Build history of the part. All positions in model axes, mm. A direction names the side the tool comes from. Give positions to 0.01 mm unless a question says otherwise; leave off trailing zeros. Order: outer loops, then holes, each group sorted by start corner. A loop starts at its lowest first (then second) coordinate and runs counter-clockwise, first axis right, second up. Notation, with made-up numbers: (84, -39) - (123, -39) arc R18 ccw to (123, -6) - close; hole circle Ø11 at (43, 70.5). An arc over 180 degrees is marked (long way). Use a Markdown table: item, result. Add a question column.
(1) Flat gauge pins, fed straight in: pin 1 (4 mm diameter, centred on y = 16.5, z = 25, fed in from -X); pin 2 (8 mm diameter, centred on x = 24.73, z = 80, fed in from +Y); pin 3 (11.5 mm diameter, centred on x = 24.73, z = 10, fed in from +Y); pin 4 (4 mm diameter, centred on x = -24.73, z = 10, fed in from -Y). Where does each tip first touch, or does it go through?
(2) Slice it at B-B (z = 31.5). Write the cut outline in (x, y), then the cut area to 3 significant figures.
(3) Wall check: line 1 (Z direction, x = -26, y = 11.5); line 2 (X direction, y = 24, z = 5); line 3 (X direction, y = 21.75, z = 5). Give the ranges that are in metal, low to high.
(4) Slice it at C-C (y = 8.5). Write the cut outline in (x, z).
(5) Which spindle directions (+Z, -Z, +X, -X, +Y, -Y) get a long thin tool onto all of the face, cutting with end or side? Do faces 4 (the face through (0, 19, 0)), 5 (the face through (-19.77, 11.97, 80.65)), 6 (the face through (-12.5, 19, 45)). Say none if no direction does.
(6) Slice it at D-D (z = 10). Write the cut outline in (x, y), then the cut area to 3 significant figures.
(7) Slice it at A-A (x = 0). Write the cut outline in (y, z).
(8) Mould opens along X. For faces 1 (the face through (-27.767, 15.397, 44.37)), 2 (the face through (22.6, 4, 77.8)), 3 (the face through (27.966, 15.032, 44.37)) say: +X half, -X half, draft (parallel to the pull), parting line (faces both ways), or undercut.
from build123d import *

# Parameters (mm, degrees)
BOSS_EXTRUDE1_DEPTH             = 90
F_5_0MM_CLEARANCE_DOWEL_HOLE1_D = 5
CUT_EXTRUDE1_REACH              = 101.384
CUT_EXTRUDE1_END_RADIUS         = 31.75
SKETCH4_R                       = 5
CUT_EXTRUDE3_DEPTH              = 101.5739779
CUT_EXTRUDE4_REACH              = 100.691
TAP_DRILL_FOR_M5X0_8_TAP1_D     = 4.2
TAP_DRILL_FOR_M5X0_8_TAP1_DEPTH = 8
TAP_DRILL_FOR_M5X0_8_TAP1_TIP   = 1.2618073


with BuildPart() as part:
    # Sketch1 → Boss-Extrude1 (new body)
    with BuildSketch(Plane.XY):
        with BuildLine():
            Line((-31.734248061, 1), (-17.721808598, 1))
            ThreePointArc((-17.721808598, 1), (0, 17.75), (17.721808598, 1))
            Line((17.721808598, 1), (31.734248061, 1))
            ThreePointArc((31.734248061, 1), (0, 31.75), (-31.734248061, 1))
        make_face()
    extrude(amount=BOSS_EXTRUDE1_DEPTH)

    # Ø5.0mm Clearance Dowel Hole1 (through all)
    with Locations(Plane(origin=(-24.72802833, 1, 80), x_dir=(0, 0, -1), z_dir=(0, -1, 0))):
        with Locations((0, 0), (70, 0), (0, 49.45605666), (70, 49.45605666)):
            Hole(F_5_0MM_CLEARANCE_DOWEL_HOLE1_D / 2)

    # Cut-Extrude1: up to this cylinder (the profile starts inside it)
    cut_extrude1_end = Plane(origin=(0, 0, 45), z_dir=(0, 0, -1)) * Cylinder(CUT_EXTRUDE1_END_RADIUS, 337.268, mode=Mode.PRIVATE)
    # Sketch4 → Cut-Extrude1 (cut, up to the surface)
    with BuildSketch(Plane(origin=(0, 4, 0), x_dir=(-1, 0, 0), z_dir=(0, -1, 0)), mode=Mode.PRIVATE) as cut_extrude1_sk1:
        with Locations(Location((24.72802833, -80, 0), (0, 0, 90))):
            Circle(SKETCH4_R)
    cut_extrude1_tool1 = extrude(cut_extrude1_sk1.sketch, amount=-CUT_EXTRUDE1_REACH, mode=Mode.PRIVATE) & cut_extrude1_end
    add(cut_extrude1_tool1.solids().sort_by_distance((-24.728028, 4, 80))[0], mode=Mode.SUBTRACT)
    # Sketch4 → Cut-Extrude1 (cut, up to the surface)
    with BuildSketch(Plane(origin=(0, 4, 0), x_dir=(-1, 0, 0), z_dir=(0, -1, 0)), mode=Mode.PRIVATE) as cut_extrude1_sk2:
        with Locations(Location((24.72802833, -10, 0), (0, 0, 90))):
            Circle(SKETCH4_R)
    cut_extrude1_tool2 = extrude(cut_extrude1_sk2.sketch, amount=-CUT_EXTRUDE1_REACH, mode=Mode.PRIVATE) & cut_extrude1_end
    add(cut_extrude1_tool2.solids().sort_by_distance((-24.728028, 4, 10))[0], mode=Mode.SUBTRACT)
    # Sketch4 → Cut-Extrude1 (cut, up to the surface)
    with BuildSketch(Plane(origin=(0, 4, 0), x_dir=(-1, 0, 0), z_dir=(0, -1, 0)), mode=Mode.PRIVATE) as cut_extrude1_sk3:
        with Locations(Location((-24.72802833, -10, 0), (0, 0, 90))):
            Circle(SKETCH4_R)
    cut_extrude1_tool3 = extrude(cut_extrude1_sk3.sketch, amount=-CUT_EXTRUDE1_REACH, mode=Mode.PRIVATE) & cut_extrude1_end
    add(cut_extrude1_tool3.solids().sort_by_distance((24.728028, 4, 10))[0], mode=Mode.SUBTRACT)
    # Sketch4 → Cut-Extrude1 (cut, up to the surface)
    with BuildSketch(Plane(origin=(0, 4, 0), x_dir=(-1, 0, 0), z_dir=(0, -1, 0)), mode=Mode.PRIVATE) as cut_extrude1_sk4:
        with Locations(Location((-24.72802833, -80, 0), (0, 0, 90))):
            Circle(SKETCH4_R)
    cut_extrude1_tool4 = extrude(cut_extrude1_sk4.sketch, amount=-CUT_EXTRUDE1_REACH, mode=Mode.PRIVATE) & cut_extrude1_end
    add(cut_extrude1_tool4.solids().sort_by_distance((24.728028, 4, 80))[0], mode=Mode.SUBTRACT)

    # Sketch8 → Cut-Extrude3 (cut, through all)
    with BuildSketch(Plane.XY.offset(90)):
        with BuildLine():
            Line((18, 26.154588508), (-18, 26.154588508))
            ThreePointArc((-18, 26.154588508), (0, 31.75), (18, 26.154588508))
        make_face()
    extrude(amount=-CUT_EXTRUDE3_DEPTH, mode=Mode.SUBTRACT)

    # Sketch9 → Cut-Extrude4 (cut, up to next)
    with BuildSketch(Plane.XZ.offset(-1), mode=Mode.PRIVATE) as cut_extrude4_sk1:
        with BuildLine():
            Line((-12.5, 25), (-12.5, 65))
            ThreePointArc((-12.5, 65), (0, 77.5), (12.5, 65))
            Line((12.5, 65), (12.5, 25))
            ThreePointArc((12.5, 25), (0, 12.5), (-12.5, 25))
        make_face()
    cut_extrude4_tool1 = extrude(cut_extrude4_sk1.sketch, amount=-CUT_EXTRUDE4_REACH, mode=Mode.PRIVATE) & part.part
    add(cut_extrude4_tool1.solids().sort_by_distance((0, 1, 45))[0], mode=Mode.SUBTRACT)

    # Tap Drill for M5x0.8 Tap1
    with Locations(Plane(origin=(-12.5, 26.154588508, 5), x_dir=(0, 0, 1), z_dir=(0, 1, 0))):
        with Locations((0, 0), (0, 25), (80, 25), (80, 0)):
            Hole(TAP_DRILL_FOR_M5X0_8_TAP1_D / 2, depth=TAP_DRILL_FOR_M5X0_8_TAP1_DEPTH)
            with Locations((0, 0, -(TAP_DRILL_FOR_M5X0_8_TAP1_DEPTH + TAP_DRILL_FOR_M5X0_8_TAP1_TIP / 2))):  # 118° drill point
                Cone(0, TAP_DRILL_FOR_M5X0_8_TAP1_D / 2, TAP_DRILL_FOR_M5X0_8_TAP1_TIP, mode=Mode.SUBTRACT)


solid = part.part
Solution:
| question | item | result |
|---|---|---|
| 1 | pin 1 | x = -28.25 |
| 1 | pin 2 | y = 4 |
| 1 | pin 3 | y = 25.45 |
| 1 | pin 4 | through |
| 2 | outline | (-31.73, 1) - (-17.72, 1) arc R17.75 cw to (-12.5, 12.6) - (-12.5, 26.15) - (-18, 26.15) arc R31.75 ccw to start; (12.5, 12.6) arc R17.75 cw to (17.72, 1) - (31.73, 1) arc R31.75 ccw to (18, 26.15) - (12.5, 26.15) - close |
| 2 | area | 674 mm2 |
| 3 | line 1 | 0 to 5.16, 14.84 to 75.16, 84.84 to 90 |
| 3 | line 2 | -20.79 to -14.6, -10.4 to 10.4, 14.6 to 20.79 |
| 3 | line 3 | -23.13 to -14.6, -10.4 to 10.4, 14.6 to 23.13 |
| 4 | outline | (-30.59, 0) - (-15.58, 0) - (-15.58, 90) - (-30.59, 90) - close; (15.58, 0) - (30.59, 0) - (30.59, 90) - (15.58, 90) - close; hole circle Ø10 at (-24.73, 10); hole circle Ø10 at (-24.73, 80); hole circle Ø10 at (24.73, 10); hole circle Ø10 at (24.73, 80) |
| 5 | face 4 | -Z, +X, -X, +Y, -Y |
| 5 | face 5 | +Y |
| 5 | face 6 | +Y, -Y |
| 6 | outline | (-31.73, 1) - (-27.23, 1) - (-27.23, 4) - (-29.73, 4) - (-29.73, 11.15) arc R31.75 ccw to start; (-22.23, 1) - (-17.72, 1) arc R17.75 cw to (17.72, 1) - (22.23, 1) - (22.23, 4) - (19.73, 4) - (19.73, 24.88) arc R31.75 ccw to (18, 26.15) - (-18, 26.15) arc R31.75 ccw to (-19.73, 24.88) - (-19.73, 4) - (-22.23, 4) - close; (27.23, 1) - (31.73, 1) arc R31.75 ccw to (29.73, 11.15) - (29.73, 4) - (27.23, 4) - close |
| 6 | area | 587 mm2 |
| 7 | outline | (17.75, 0) - (26.15, 0) - (26.15, 12.5) - (17.75, 12.5) - close; (17.75, 77.5) - (26.15, 77.5) - (26.15, 90) - (17.75, 90) - close |
| 8 | face 1 | -X half |
| 8 | face 2 | undercut |
| 8 | face 3 | +X half |
